Verification items for the finished model (mm, model axes). A direction names the side the tool comes from. Coordinates: 2 decimals unless noted, no trailing zeros. Order: outer loops, then holes, each group sorted by start corner. A loop starts at its lowest first (then second) coordinate and runs counter-clockwise, first axis right, second up. Notation, with made-up numbers: M -15.5,-23 L 43.5,-23 A24 cw 43.5,4 Z; hole C 84,-4 d9. An arc over 180 degrees is marked long. Write item = value, one per line.
```python
from build123d import *

# Parameters (mm, degrees)
SKETCH_R        = 1.6
PAD_DEPTH       = 5
SKETCH001_R     = 1.6
POCKET_DEPTH    = 5.001
SKETCH002_R     = 3
POCKET001_DEPTH = 3


with BuildPart() as part:
    # Sketch → Pad (new body, symmetric)
    with BuildSketch(Plane.XZ):
        Polygon((11, 5), (11, 0), (3.5, 0), (3.5, 2), (-3.5, 2), (-3.5, 0), (-11, 0), (-11, 5), (-4, 5), (-4, 14), (4, 14), (4, 5), align=None)
        with Locations((0, 10.8)):
            Circle(SKETCH_R, mode=Mode.SUBTRACT)
    extrude(amount=PAD_DEPTH, both=True)

    # Sketch001 (on DatumPlane) → Pocket (cut, through all)
    with BuildSketch(Plane.XY.offset(5)):
        with Locations((-7, 0)):
            Circle(SKETCH001_R)
        with Locations((7, 0)):
            Circle(SKETCH001_R)
    extrude(amount=-POCKET_DEPTH, mode=Mode.SUBTRACT)

    # Sketch002 (on DatumPlane) → Pocket001 (cut)
    with BuildSketch(Plane.XY.offset(5)):
        with Locations((-7, 0)):
            Circle(SKETCH002_R)
        with Locations((7, 0)):
            Circle(SKETCH002_R)
    extrude(amount=-POCKET001_DEPTH, mode=Mode.SUBTRACT)


solid = part.part
```
Item 1: Sectioned sample at A-A, the plane x = 0. Enter the section's corners in (y, z), then the cut area to 3 significant figures.
Report:
outline = M -5,2 L 5,2 L 5,9.2 L -5,9.2 Z; M -5,12.4 L 5,12.4 L 5,14 L -5,14 Z
area = 88.0 mm^2
Item 2: Sectioned sample at B-B, the plane z = 10.8. Enter the section's corners in (x, y).
Report:
outline = M -4,-5 L -1.6,-5 L -1.6,5 L -4,5 Z; M 1.6,-5 L 4,-5 L 4,5 L 1.6,5 Z
Item 3: Scan lines: L1, parallel to X at y = -2.25, z = 4; L2, parallel to Y at x = 7, z = 3.35; L3, parallel to X at y = 2, z = 7.75. Record each from-to range of solid material in increasing order. Write a range as from..to.
Report:
L1 = -11..-8.98, -5.02..5.02, 8.98..11
L2 = -5..-3, 3..5
L3 = -4..4
Item 4: Tool access check on faces 1 (the flat face through (3.5, 0, 1)), 2 (the flat face through (4, 0, 10)), 3 (the flat face through (-4, 0, 9)). Record the directions out of +Z, -Z, +X, -X, +Y, -Y that give a thin tool (end or side, any length) a straight path to the whole face; none if there is none.
Report:
face_1 = -Z, +Y, -Y
face_2 = +Z, +X, +Y, -Y
face_3 = +Z, -X, +Y, -Y
Item 5: Release check for a two-part mould opening along Y. For faces 4 (the flat face through (-5.7, -1.3, 2)), 5 (the flat face through (8.3, -1.3, 2)), 6 (the flat face through (0, 5, 6)), 7 (the flat face through (-10, 1, 5)) record: pulls with the +Y half, pulls with the -Y half, needs draft (parallel to the pull), parting line crosses it, or undercut.
Report:
face_4 = undercut
face_5 = undercut
face_6 = pulls with the +Y half
face_7 = needs draft
Item 6: Gauge pin test, flat ends, axial feed: pin 1 (5 mm diameter, centred on x = 7, y = 0, fed in from +Z); pin 2 (4.5 mm diameter, centred on y = 1.5, z = 7.5, fed in from -X); pin 3 (5.5 mm diameter, centred on x = 9, y = -2, fed in from +Z). Record the tip position at first contact, or that the pin passes through.
Report:
pin_1 = 2
pin_2 = -4
pin_3 = 5
Item 7: Sectioned sample at C-C, the plane y = -3.75. Enter the section's corners in (x, z).
Report:
outline = M -11,0 L -3.5,0 L -3.5,2 L 3.5,2 L 3.5,0 L 11,0 L 11,5 L 4,5 L 4,14 L -4,14 L -4,5 L -11,5 Z; hole C 0,10.8 d3.2
Item 8: Sectioned sample at D-D, the plane z = 2.5. Enter the section's corners in (x, y).
Report:
outline = M -11,-5 L 11,-5 L 11,5 L -11,5 Z; hole C -7,0 d6; hole C 7,0 d6
